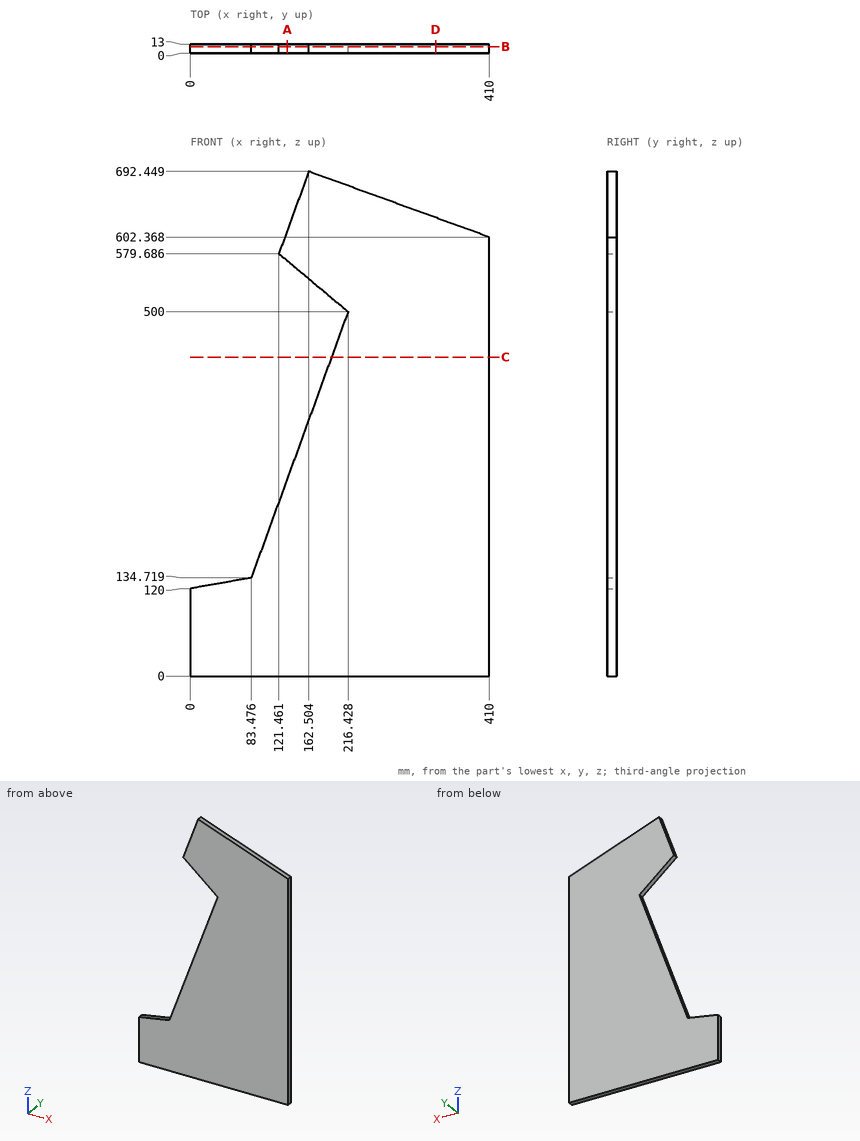
Here's the drawing with two shaded views (mm, measured from the low corner). I have some questions. Round coordinates to 2 decimals unless told otherwise and drop trailing zeros. Loops run counter-clockwise (first coordinate to the right, second up) from the corner with the lowest first, then second, coordinate; pieces in that order, holes last. Notation, with made-up numbers: M -28.5,69.5 L -3.5,69.5 A13 ccw -3.5,85.5 Z; hole C -31.75,2.25 d6. An arc over 180 degrees is marked long. Answer as a JSON object with one key per item and string values. Group by question number.
Q1. Imagine slicing it at C-C, the plane z = 437.5. Please give me the cut outline in (x, y), then the cut area to 3 significant figures.
Q2. Imagine slicing it at D-D, the plane x = 336.5. Please give me the cut outline in (y, z), then the cut area to 3 significant figures.
Q3. Imagine slicing it at B-B, the plane y = 9.25. Please give me the cut outline in (x, z).
Q4. Imagine slicing it at A-A, the plane x = 133. Please give me the cut outline in (y, z) (1 decimal), then the cut area to 3 significant figures.
Q5. Will these pins go through, and if not, where does the flat tip stop? pin 1 (4 mm diameter, centred on x = 176, y = 6, fed in from +Z) (1 decimal); pin 2 (2 mm diameter, centred on x = 359.5, y = 6, fed in from +Z).
Q6. Please list where these lines run through material, in increasing order: L1, parallel to X at y = 5.5, z = 360; L2, parallel to Z at x = 37.5, y = 8; L3, parallel to Z at x = 30, y = 4.5.
Findings:
{
 "1": {"outline": "M 193.68,0 L 410,0 L 410,13 L 193.68,13 Z", "area": "2,810 mm2"},
 "2": {"outline": "M 0,0 L 13,0 L 13,629.12 L 0,629.12 Z", "area": "8,180 mm2"},
 "3": {"outline": "M 0,0 L 410,0 L 410,602.37 L 162.5,692.45 L 121.46,579.69 L 216.43,500 L 83.48,134.72 L 0,120 Z"},
 "4": {"outline": "M 0,0 L 13,0 L 13,270.8 L 0,270.8 Z; M 0,570 L 13,570 L 13,611.4 L 0,611.4 Z", "area": "4,060 mm2"},
 "5": {"pin 1": "stops at z = 688.3", "pin 2": "stops at z = 621.11"},
 "6": {"L1": "x = 165.47 to 410", "L2": "z = 0 to 126.61", "L3": "z = 0 to 125.29"}
}
